The figure shows three views and two pictorial views of one solid part (mm, origin at its lowest corner). Answer the questions. Round coordinates to 2 decimals unless told otherwise and drop trailing zeros. Order: outer loops, then holes, each group sorted by start corner. A loop starts at its lowest first (then second) coordinate and runs counter-clockwise, first axis right, second up. Notation, with made-up numbers: (74, 52) - (133, 52) arc R33 ccw to (133, 81) - close; hole circle Ø7 at (-38.5, 69). An arc over 180 degrees is marked (long way). Answer as a JSON object with one key per item and string values. Group by question number.
Q1. Given pin 1 Ø10.5 at (x, z) = (25.4, 25.4) entering from -Y (1 decimal); pin 2 Ø20.5 at (x, z) = (25.4, 25.4) entering from +Y; pin 3 Ø2 at (y, z) = (12, 8) entering from -X (1 decimal); pin 4 Ø6 at (y, z) = (11.5, 40.5) entering from -X, each flat-ended and moving along its own axis, determine where each tip first touches the part or whether it passes through.
Q2. Consider line 1 (Z direction, x = 25.4, y = 5.3); line 2 (Z direction, x = 25.4, y = 8.5); line 3 (X direction, y = 11, z = 26). Determine where each line is inside the solid, lowest interval first.
Q3. A cutting plane is placed at A-A on y = 1.5. Determine the outline of the cut face in (x, z) (1 decimal), and give its area (3 significant figures).
Q4. A cutting plane is placed at B-B on y = 9.75. Determine the outline of the cut face in (x, z), and give its area (3 significant figures).
Q5. The mould has two halves that part along X. Classify the marked faces 1, 2 and 3: pulls with the +X half, pulls with the -X half, needs draft (parallel to the pull), parting line crosses it, or undercut.
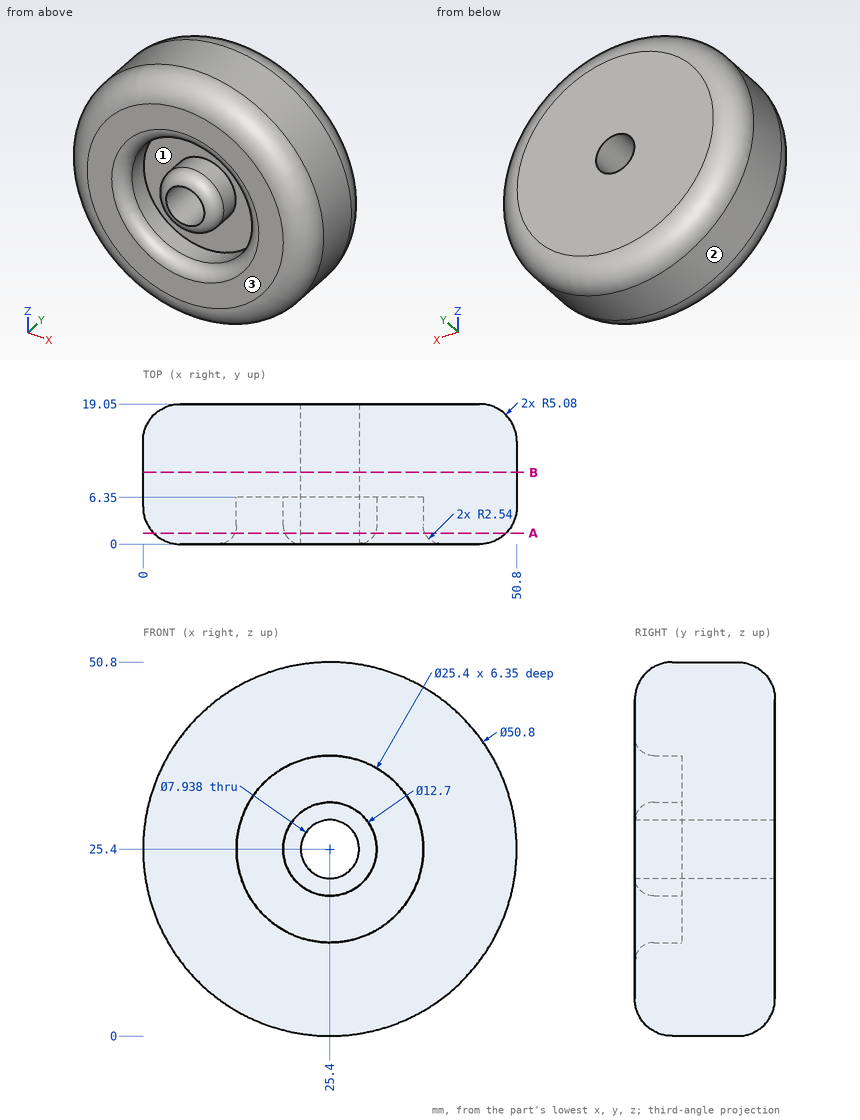
Result set:
{
 "1": {"pin 1": "stops at y = 0", "pin 2": "stops at y = 19.05", "pin 3": "stops at x = 6", "pin 4": "stops at x = 3.07"},
 "2": {"line 1": "z = 0 to 12.7, 19.05 to 21.43, 29.37 to 31.75, 38.1 to 50.8", "line 2": "z = 0 to 21.43, 29.37 to 50.8", "line 3": "x = 0.01 to 21.48, 29.32 to 50.79"},
 "3": {"outline": "circle Ø47.8 at (25.4, 25.4); circle Ø12.3 at (25.4, 25.4); hole circle Ø25.8 at (25.4, 25.4); hole circle Ø7.9 at (25.4, 25.4)", "area": "1,340 mm²"},
 "4": {"outline": "circle Ø50.8 at (25.4, 25.4); hole circle Ø7.94 at (25.4, 25.4)", "area": "1,980 mm²"},
 "5": {"face 1": "undercut", "face 2": "parting line crosses it", "face 3": "needs draft"}
}
